Can you work these out from the model? Positions are in its coordinate system, mm. A direction names the side the tool comes from. Give positions to 0.01 mm unless a question says otherwise; leave off trailing zeros. Order: outer loops, then holes, each group sorted by start corner. A loop starts at its lowest first (then second) coordinate and runs counter-clockwise, first axis right, second up. Notation, with made-up numbers: (29, 74.25) - (87, 74.25) arc R29 cw to (87, 102.25) - close; hole circle Ø3 at (8.25, 77). An arc over 180 degrees is marked (long way). Return JSON: item names as keys, results as strings.
```python
from build123d import *

# Parameters (mm, degrees)
SKETCH_W        = 46
SKETCH_H        = 48
PAD_DEPTH       = 10
SKETCH001_R     = 1.5
POCKET_DEPTH    = 46.001
SKETCH002_R     = 1.6
POCKET001_DEPTH = 10.001
PAD001_DEPTH    = 48
PAD001_FACE20_R = 1.6
POCKET002_DEPTH = 1.501
SKETCH004_W     = 9
SKETCH004_H     = 9
POCKET003_DEPTH = 1.5
FILLET_R        = 3
POCKET004_DEPTH = 10.5


with BuildPart() as part:
    # Sketch → Pad (new body)
    with BuildSketch(Plane.XY):
        with Locations((-3, 0)):
            Rectangle(SKETCH_W, SKETCH_H)
        with BuildLine():
            ThreePointArc((-5, 11), (-13, 19), (-21, 11))
            Line((-21, 11), (-21, -11))
            ThreePointArc((-21, -11), (-13, -19), (-5, -11))
            Line((-5, 11), (-5, -11))
        make_face(mode=Mode.SUBTRACT)
    extrude(amount=PAD_DEPTH)

    # Sketch001 (on Face2 of Pad) → Pocket (cut, through all)
    with BuildSketch(Plane(origin=(-26, 0, 0), x_dir=(0, -1, 0), z_dir=(-1, 0, 0))):
        with Locations((-15.8, 5)):
            Circle(SKETCH001_R)
        with Locations((15.8, 5)):
            Circle(SKETCH001_R)
    extrude(amount=-POCKET_DEPTH, mode=Mode.SUBTRACT)

    # Sketch002 (on Face5 of Pocket) → Pocket001 (cut, through all)
    with BuildSketch(Plane.XY.offset(10)):
        with Locations((10, 10)):
            Circle(SKETCH002_R)
        with Locations((10, -10)):
            Circle(SKETCH002_R)
    extrude(amount=-POCKET001_DEPTH, mode=Mode.SUBTRACT)

    # Sketch003 (on Face1 of Pocket001) → Pad001 (join)
    with BuildSketch(Plane(origin=(0, 24, 0), x_dir=(-1, 0, 0), z_dir=(0, 1, 0))):
        Polygon((-12.75, 11.5), (-7.25, 11.5), (-5.5, 10), (-14.5, 10), align=None)
    extrude(amount=-PAD001_DEPTH)

    # Pad001 Face20 → Pocket002 (cut, through all)
    with BuildSketch(Plane(origin=(10, 10, 10), x_dir=(0, -1, 0), z_dir=(0, 0, -1))):
        Circle(PAD001_FACE20_R)
    extrude(amount=-POCKET002_DEPTH, mode=Mode.SUBTRACT)

    # Sketch004 (on Face10 of Pocket002) → Pocket003 (cut)
    with BuildSketch(Plane.XY.offset(11.5)):
        with Locations((10, 10)):
            Rectangle(SKETCH004_W, SKETCH004_H)
        with Locations((10, -10)):
            Rectangle(SKETCH004_W, SKETCH004_H)
    extrude(amount=-POCKET003_DEPTH, mode=Mode.SUBTRACT)

    # Fillet
    fillet_edges = [part.edges().sort_by_distance(p)[0] for p in [
        (-26, -24, 5),
        (-26, 24, 5),
        (20, -24, 5),
        (20, 24, 5),
    ]]
    fillet(fillet_edges, radius=FILLET_R)

    # Sketch006 (on Face1 of Fillet) → Pocket004 (cut)
    with BuildSketch(Plane.YZ.offset(20)):
        Polygon((-12.624574, 5), (-14.212287, 7.75), (-17.387713, 7.75), (-18.975426, 5), (-17.387713, 2.25), (-14.212287, 2.25), align=None)
        Polygon((17.387713, 7.75), (14.212287, 7.75), (12.624574, 5), (14.212287, 2.25), (17.387713, 2.25), (18.975426, 5), align=None)
    extrude(amount=-POCKET004_DEPTH, mode=Mode.SUBTRACT)


solid = part.part
```
1. Suppose I cut it at D-D (x = -9). List the corners of the cut face in (y, z) for me, plus the area to 3 significant figures.
Checks:
{"outline": "(-24, 0) - (-17.93, 0) - (-17.93, 10) - (-24, 10) - close; (17.93, 0) - (24, 0) - (24, 10) - (17.93, 10) - close", "area": "121 mm^2"}
2. On a 3-axis mill with a long thin cutter (end or side, diameter ignored), from which of +Z, -Z, +X, -X, +Y, -Y can I reach the whole of each face in a straight line? I mean faces 4 (the face through (10, -5.5, 11)), 5 (the face through (15, 16, 7.75)), 6 (the face through (-13, -19, 5)). Say none if no direction works.
Checks:
{"face 4": "+Z, +X, -X", "face 5": "+X", "face 6": "+Z, -Z"}
3. If I drill on L1, parallel to Z at x = -22, y = -15.8; L2, parallel to X at y = 10, z = 5.75; L3, parallel to X at y = -1, z = 1.5, over which ranges is the centre line in solid material (lowest first)? Write a range as [from, to].
Checks:
{"L1": "[0, 3.5], [6.5, 10]", "L2": "[-26, -21], [-5, 8.4], [11.6, 20]", "L3": "[-26, -21], [-5, 20]"}
4. Thinking about a two-plate mould opening in X: for faces 1 (the face through (-21, 0, 5)), 2 (the face through (2, 0, 0)), 3 (the face through (6.387, -19.184, 10.76)), which applies, +X half, -X half, draft (parallel to the pull), parting line (faces both ways), or undercut?
Checks:
{"face 1": "undercut", "face 2": "draft", "face 3": "-X half"}
5. Suppose I cut it at C-C (y = 10). List the corners of the cut face in (x, z) for me.
Checks:
{"outline": "(-26, 0) - (-21, 0) - (-21, 10) - (-26, 10) - close; (-5, 0) - (8.4, 0) - (8.4, 10) - (-5, 10) - close; (11.6, 0) - (20, 0) - (20, 10) - (11.6, 10) - close"}
6. For pin 1 Ø14 at (x, y) = (-9.5, 3) entering from +Z; pin 2 Ø3 at (y, z) = (-15, 5.5) entering from +X; pin 3 Ø1.9 at (x, y) = (10, -10) entering from -Z, each with a flat end and sliding along its axis, tell me the tip position at first contact or that it passes through.
Checks:
{"pin 1": "z = 10", "pin 2": "x = 9.5", "pin 3": "through"}
7. Suppose I cut it at B-B (z = 9). List the corners of the cut face in (x, y) for me, plus the area to 3 significant figures.
Checks:
{"outline": "(-26, -21) arc R3 ccw to (-23, -24) - (17, -24) arc R3 ccw to (20, -21) - (20, 21) arc R3 ccw to (17, 24) - (-23, 24) arc R3 ccw to (-26, 21) - close; hole (-21, -11) arc R8 ccw to (-5, -11) - (-5, 11) arc R8 ccw to (-21, 11) - close; hole circle Ø3.2 at (10, -10); hole circle Ø3.2 at (10, 10)", "area": "1,630 mm^2"}
8. Suppose I cut it at A-A (y = 15.8). List the corners of the cut face in (x, z) for me, plus the area to 3 significant figures.
Checks:
{"outline": "(-26, 0) - (-19.4, 0) - (-19.4, 3.5) - (-26, 3.5) - close; (-26, 6.5) - (-19.4, 6.5) - (-19.4, 10) - (-26, 10) - close; (-6.6, 0) - (20, 0) - (20, 2.25) - (9.5, 2.25) - (9.5, 3.5) - (-6.6, 3.5) - close; (-6.6, 6.5) - (9.5, 6.5) - (9.5, 7.75) - (20, 7.75) - (20, 10) - (14.5, 10) - (12.75, 11.5) - (7.25, 11.5) - (5.5, 10) - (-6.6, 10) - close", "area": "217 mm^2"}
